from build123d import *

# Parameters (mm, degrees)
SKETCH2_W           = 16.400211148
SKETCH2_H           = 13
BOSS_EXTRUDE1_DEPTH = 3
SKETCH3_W           = 16.430845556
SKETCH3_H           = 2.401527161
SKETCH3_H_2         = 2.320561052
CUT_EXTRUDE1_DEPTH  = 3
SKETCH4_R           = 2
CUT_EXTRUDE2_DEPTH  = 3
SKETCH5_W           = 15
SKETCH5_H           = 15
BOSS_EXTRUDE3_DEPTH = 18
SKETCH6_W           = 13
SKETCH6_H           = 13
CUT_EXTRUDE3_DEPTH  = 20
SKETCH7_R           = 2
CUT_EXTRUDE4_DEPTH  = 5


with BuildPart() as part:
    # Sketch1 → Revolve1 (revolve)
    with BuildSketch(Plane.XY, mode=Mode.PRIVATE) as revolve1_sk:
        with BuildLine():
            Line((10, 25.165087569), (10, 5.165087569))
            ThreePointArc((10, 5.165087569), (7.071067812, -1.905980243), (0, -4.834912431))
            Line((0, -4.834912431), (0, -9.834912431))
            Line((0, -9.834912431), (0, -11.124312847))
            Line((0, -11.124312847), (8.247604153, -11.124312847))
            Line((8.247604153, -11.124312847), (8.247604153, -8.124312847))
            Line((8.247604153, -8.124312847), (2, -8.124312847))
            Line((2, -8.124312847), (2, -7.680145009))
            ThreePointArc((2, -7.680145009), (9.874208829, -3.290679693), (13, 5.165087569))
            Line((13, 5.165087569), (13, 28.165087569))
            Line((13, 28.165087569), (10, 28.165087569))
            Line((10, 28.165087569), (10, 25.165087569))
        make_face()
    revolve(revolve1_sk.sketch.rotate(Axis((0, 0, 0), (0, 1, 0)), 90), axis=Axis((0, 0, 0), (0, 1, 0)))

    # Sketch2 → Boss-Extrude1 (add)
    with BuildSketch(Plane.XZ.offset(11.124312847)):
        Rectangle(SKETCH2_W, SKETCH2_H)
    extrude(amount=-BOSS_EXTRUDE1_DEPTH)

    # Sketch3 → Cut-Extrude1 (cut)
    with BuildSketch(Plane.XZ.offset(11.124312847)):
        with Locations((0.015317204, 7.700763581)):
            Rectangle(SKETCH3_W, SKETCH3_H)
        with Locations((0.015317204, -7.704987868)):
            Rectangle(SKETCH3_W, SKETCH3_H_2)
    extrude(amount=-CUT_EXTRUDE1_DEPTH, mode=Mode.SUBTRACT)

    # Sketch4 → Cut-Extrude2 (cut)
    with BuildSketch(Plane.XZ.offset(11.124312847)):
        with Locations(Location((5, 0, 0), (0, 0, 270))):
            Circle(SKETCH4_R)
        with Locations(Location((-5, 0, 0), (0, 0, 270))):
            Circle(SKETCH4_R)
    extrude(amount=-CUT_EXTRUDE2_DEPTH, mode=Mode.SUBTRACT)

    # Sketch5 → Boss-Extrude3 (add)
    with BuildSketch(Plane(origin=(8.200105574, 0, 0), x_dir=(0, 0, -1), z_dir=(1, 0, 0))):
        with Locations((0, -15.624312847)):
            Rectangle(SKETCH5_W, SKETCH5_H)
    extrude(amount=-BOSS_EXTRUDE3_DEPTH)

    # Sketch6 → Cut-Extrude3 (cut)
    with BuildSketch(Plane.ZY.offset(9.799894426)):
        with Locations((0, -15.624312847)):
            Rectangle(SKETCH6_W, SKETCH6_H)
    extrude(amount=-CUT_EXTRUDE3_DEPTH, mode=Mode.SUBTRACT)

    # Sketch7 → Cut-Extrude4 (cut)
    with BuildSketch(Plane.XZ.offset(23.124312847)):
        with Locations(Location((-5, 0, 0), (0, 0, 270))):
            Circle(SKETCH7_R)
        with Locations(Location((5, 0, 0), (0, 0, 270))):
            Circle(SKETCH7_R)
    extrude(amount=-CUT_EXTRUDE4_DEPTH, mode=Mode.SUBTRACT)


solid = part.part
For this review, take the finished solid that the model builds, in its own axes (mm). A direction names the side the tool comes from. Coordinates: 2 decimals unless noted, no trailing zeros. Order: outer loops, then holes, each group sorted by start corner. A loop starts at its lowest first (then second) coordinate and runs counter-clockwise, first axis right, second up. Notation, with made-up numbers: (67.25, 14.5) -> (116.25, 14.5) arc R17 ccw to (116.25, 18.5) -> close; hole circle Ø3 at (82.5, 44.5). An arc over 180 degrees is marked (long way). Return JSON: item names as keys, results as strings.
1. Machinability: for faces 4 (the flat face through (-1, -16, -6.5)), 5 (the flat face through (-9.8, -16, 7)), 6 (the cylindrical face through (8.248, -8.617, 0.012)), 7 (the flat face through (-1, -16, -7.5)), which of the approach directions +Z, -Z, +X, -X, +Y, -Y give a long, thin tool a straight path to every point of the face, cutting with its end or side? Answer none if there is none.
Answer block:
{"face 4": "+X, -X", "face 5": "+Z, -Z, -X, -Y", "face 6": "+X, -Y", "face 7": "-Z, +X, -X, -Y"}
2. We need section B-B on x = -8.75. Write out the cut boundary in (y, z), and give its area (3 significant figures).
Answer block:
{"outline": "(-23.12, -7.5) -> (-8.12, -7.5) -> (-8.12, 7.5) -> (-23.12, 7.5) -> close; (5.17, -9.61) -> (28.17, -9.61) -> (28.17, -4.84) -> (5.17, -4.84) arc R4.84 cw to (5.17, 4.84) -> (28.17, 4.84) -> (28.17, 9.61) -> (5.17, 9.61) arc R9.61 ccw to start; hole (-22.12, -6.5) -> (-9.12, -6.5) -> (-9.12, 6.5) -> (-22.12, 6.5) -> close", "area": "384 mm²"}
3. We need section A-A on z = 0. Write out the cut boundary in (x, y).
Answer block:
{"outline": "(-13, 5.17) arc R13 ccw to (-2, -7.68) -> (-2, -8.12) -> (-9.8, -8.12) -> (-9.8, -9.12) -> (8.25, -9.12) -> (8.25, -8.12) -> (2, -8.12) -> (2, -7.68) arc R13 ccw to (13, 5.17) -> (13, 28.17) -> (10, 28.17) -> (10, 5.17) arc R10 cw to (-10, 5.17) -> (-10, 28.17) -> (-13, 28.17) -> close; (-9.8, -23.12) -> (-7, -23.12) -> (-7, -22.12) -> (-9.8, -22.12) -> close; (-3, -23.12) -> (3, -23.12) -> (3, -22.12) -> (-3, -22.12) -> close; (7, -23.12) -> (8.2, -23.12) -> (8.2, -22.12) -> (7, -22.12) -> close"}
4. The part is to be moulded in two halves that separate along X. For faces 1 (the flat face through (-1, -22.124, 0)), 2 (the cylindrical face through (6.983, -22.631, 0.26)), 3 (the cylindrical face through (1.952, -7.899, 0.434)), say which applies: +X half, -X half, draft (parallel to the pull), parting line (faces both ways), or undercut.
Answer block:
{"face 1": "draft", "face 2": "undercut", "face 3": "parting line"}
5. For pin 1 Ø6.5 at (x, z) = (2, 0.5) entering from +Y; pin 2 Ø3 at (y, z) = (-3.5, -9) entering from +X; pin 3 Ø14.5 at (x, y) = (-4.5, -13.5) entering from +Z, all flat-tipped, find the tip position at first contact; note any pin that passes through.
Answer block:
{"pin 1": "y = -3.31", "pin 2": "x = 6.94", "pin 3": "z = 7.5"}
6. For line 1 (X direction, y = -22.8, z = 0); line 2 (Y direction, x = -4.5, z = -6.25); line 3 (Y direction, x = -9.75, z = 3.5), list the stretches that pass through material, from the lowest coordinate up. Write a range as from..to.
Answer block:
{"line 1": "-9.8..-7, -3..3, 7..8.2", "line 2": "-23.12..-22.12, -9.12..-8.12, -5.31..-1.21", "line 3": "-23.12..-22.12, -9.12..-8.12, -2.69..28.17"}
7. We need section D-D on y = 13.5. Write out the cut boundary in (x, z).
Answer block:
{"outline": "circle Ø26 at (0, 0); hole circle Ø20 at (0, 0)"}
8. We need section C-C on x = 0. Write out the cut boundary in (y, z), and give its area (3 significant figures).
Answer block:
{"outline": "(-23.12, -7.5) -> (-8.12, -7.5) -> (-8.12, -2) -> (-7.68, -2) arc R13 ccw to (5.17, -13) -> (28.17, -13) -> (28.17, -10) -> (5.17, -10) arc R10 cw to (5.17, 10) -> (28.17, 10) -> (28.17, 13) -> (5.17, 13) arc R13 ccw to (-7.68, 2) -> (-8.12, 2) -> (-8.12, 7.5) -> (-23.12, 7.5) -> close; hole (-22.12, -6.5) -> (-9.12, -6.5) -> (-9.12, 6.5) -> (-22.12, 6.5) -> close", "area": "304 mm²"}
